Design review of the part built by this model. Coordinates are the model's own, in mm. Round coordinates to 2 decimals unless told otherwise and drop trailing zeros. Order: outer loops, then holes, each group sorted by start corner. A loop starts at its lowest first (then second) coordinate and runs counter-clockwise, first axis right, second up. Notation, with made-up numbers: (0.5, 83) - (5.5, 83) arc R18 ccw to (5.5, 101) - close; hole circle Ø11 at (4, 46). An arc over 180 degrees is marked (long way). Write item = value, one per line.
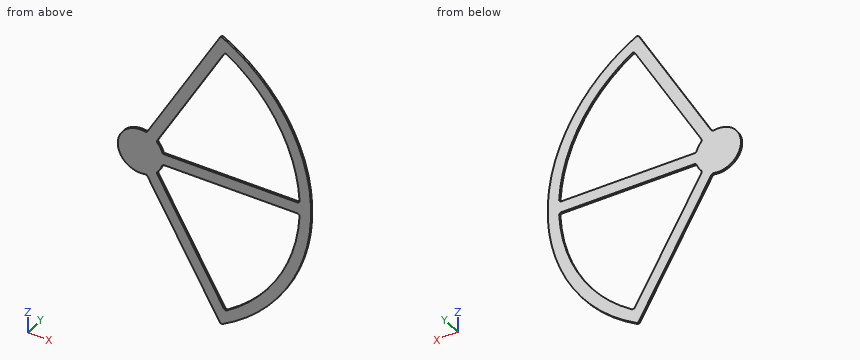
from build123d import *

# Parameters (mm, degrees)
BOSS_EXTRUDE1_DEPTH = 1.75


with BuildPart() as part:
    # Sketch1 → Boss-Extrude1 (new body)
    with BuildSketch(Plane(origin=(0, 0, 0), x_dir=(1, 0, 0), z_dir=(0, 1, 0))):
        with BuildLine():
            Line((6.098199788, 20.562391868), (69.654668716, 130.645425201))
            ThreePointArc((69.654668716, 130.645425201), (70.84952744, 131.571931019), (72.351404923, 131.397390407))
            ThreePointArc((72.351404923, 131.397390407), (150, 0), (72.351404923, -131.397390407))
            ThreePointArc((72.351404923, -131.397390407), (70.84952744, -131.571931019), (69.654668716, -130.645425201))
            Line((69.654668716, -130.645425201), (6.098199788, -20.562391868))
            ThreePointArc((6.098199788, -20.562391868), (5.188430073, -19.739247934), (3.969226346, -19.602174426))
            ThreePointArc((3.969226346, -19.602174426), (-20, 0), (3.969226346, 19.602174426))
            ThreePointArc((3.969226346, 19.602174426), (5.188430073, 19.739247934), (6.098199788, 20.562391868))
        make_face()
        with BuildLine():
            Line((20.856653615, 5), (137.822349421, 5))
            ThreePointArc((137.822349421, 5), (139.271987057, 5.622120933), (139.819774775, 7.101449275))
            ThreePointArc((139.819774775, 7.101449275), (121.24355653, 70), (76.059922864, 117.536752269))
            ThreePointArc((76.059922864, 117.536752269), (74.504893079, 117.802018361), (73.24130173, 116.857655808))
            Line((73.24130173, 116.857655808), (14.758453826, 15.562391868))
            ThreePointArc((14.758453826, 15.562391868), (14.500475126, 14.362936215), (14.991367849, 13.238538062))
            ThreePointArc((14.991367849, 13.238538062), (17.320508076, 10), (18.960594195, 6.363636364))
            ThreePointArc((18.960594195, 6.363636364), (19.688905198, 5.376311718), (20.856653615, 5))
        make_face(mode=Mode.SUBTRACT)
        with BuildLine():
            Line((20.856653615, -5), (137.822349421, -5))
            ThreePointArc((137.822349421, -5), (139.271987057, -5.622120933), (139.819774775, -7.101449275))
            ThreePointArc((139.819774775, -7.101449275), (121.24355653, -70), (76.059922864, -117.536752269))
            ThreePointArc((76.059922864, -117.536752269), (74.504893079, -117.802018361), (73.24130173, -116.857655808))
            Line((73.24130173, -116.857655808), (14.758453826, -15.562391868))
            ThreePointArc((14.758453826, -15.562391868), (14.500475126, -14.362936215), (14.991367849, -13.238538062))
            ThreePointArc((14.991367849, -13.238538062), (17.320508076, -10), (18.960594195, -6.363636364))
            ThreePointArc((18.960594195, -6.363636364), (19.688905198, -5.376311718), (20.856653615, -5))
        make_face(mode=Mode.SUBTRACT)
    extrude(amount=BOSS_EXTRUDE1_DEPTH)


solid = part.part
1) We need section A-A on z = -101. Write out the cut boundary in (x, y).
Findings:
outline = (52.54, 0) - (64.09, 0) - (64.09, 1.75) - (52.54, 1.75) - close; (96.95, 0) - (110.9, 0) - (110.9, 1.75) - (96.95, 1.75) - close
2) Clearance check with flat-ended pins moving along their axes: pin 1 Ø0.9 at (x, y) = (65, 1.5) entering from -Z; pin 2 Ø1 at (x, y) = (121.5, 1) entering from +Z. State where each tip first meets the part, or that it passes through.
Findings:
pin_1 = -123.36
pin_2 = 88.65
3) We need section B-B on x = 81. Write out the cut boundary in (y, z).
Findings:
outline = (0, -126.25) - (1.75, -126.25) - (1.75, -114.19) - (0, -114.19) - close; (0, -5) - (1.75, -5) - (1.75, 5) - (0, 5) - close; (0, 114.19) - (1.75, 114.19) - (1.75, 126.25) - (0, 126.25) - close
4) We need section C-C on y = 1.4. Write out the cut boundary in (x, z).
Findings:
outline = (3.97, -19.6) arc R2 cw to (6.1, -20.56) - (69.65, -130.65) arc R2 ccw to (72.35, -131.4) arc R150 ccw to (72.35, 131.4) arc R2 ccw to (69.65, 130.65) - (6.1, 20.56) arc R2 cw to (3.97, 19.6) arc R20 ccw (long way) to start; hole (14.76, -15.56) - (73.24, -116.86) arc R2 ccw to (76.06, -117.54) arc R140 ccw to (139.82, -7.1) arc R2 ccw to (137.82, -5) - (20.86, -5) arc R2 ccw to (18.96, -6.36) arc R20 cw to (14.99, -13.24) arc R2 ccw to start; hole (14.76, 15.56) arc R2 ccw to (14.99, 13.24) arc R20 cw to (18.96, 6.36) arc R2 ccw to (20.86, 5) - (137.82, 5) arc R2 ccw to (139.82, 7.1) arc R140 ccw to (76.06, 117.54) arc R2 ccw to (73.24, 116.86) - close
5) We need section D-D on z = -36.5. Write out the cut boundary in (x, y).
Findings:
outline = (15.3, 0) - (26.85, 0) - (26.85, 1.75) - (15.3, 1.75) - close; (135.16, 0) - (145.49, 0) - (145.49, 1.75) - (135.16, 1.75) - close
6) To check wall thickness, follow L1, parallel to Z at x = 100, y = 0.6; L2, parallel to Z at x = 70, y = 1.55; L3, parallel to X at y = 0.4, z = 112. State the ranges of each line that lie inside material, in increasing order. Write a range as from..to.
Findings:
L1 = -111.8..-97.98, -5..5, 97.98..111.8
L2 = -131.09..-111.24, -5..5, 111.24..131.09
L3 = 58.89..70.44, 84..99.78
